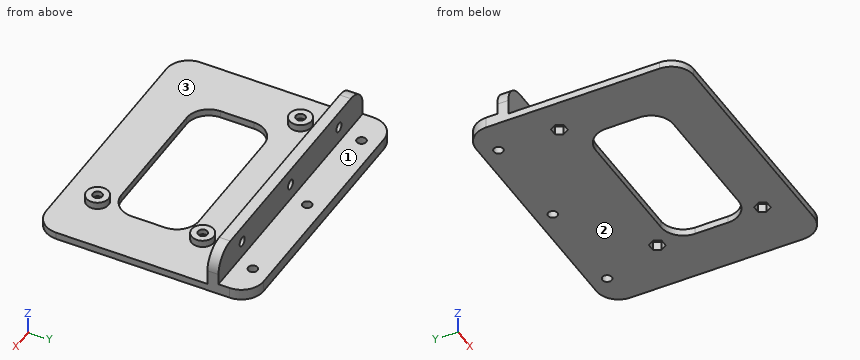
```python
from build123d import *

# Parameters (mm, degrees)
F0_W     = 121.6
F0_H     = 78.3
F0_R     = 2.125
F1_DEPTH = 3.2
F2_R     = 5
F2_R_2   = 2.125
F3_DEPTH = 3.2
F5_DEPTH = 4
F6_W     = 121.6
F6_H     = 20
F6_R     = 2.125
F7_DEPTH = 5
F8_W     = 121.6
F8_H     = 15
F8_R     = 2.125
F9_DEPTH = 5
F10_R    = 10


with BuildPart() as f1:
    # F0 (on Top) → F1 (new body)
    with BuildSketch(Plane.XY):
        Rectangle(F0_W, F0_H)
        with Locations((35.5, -24.05)):
            Circle(F0_R, mode=Mode.SUBTRACT)
        with BuildLine():
            ThreePointArc((37.5, -7.5), (34.571068, -14.571068), (27.5, -17.5))
            Line((27.5, -17.5), (-27.5, -17.5))
            ThreePointArc((-27.5, -17.5), (-34.571068, -14.571068), (-37.5, -7.5))
            Line((-37.5, -7.5), (-37.5, 7.5))
            ThreePointArc((-37.5, 7.5), (-34.571068, 14.571068), (-27.5, 17.5))
            Line((-27.5, 17.5), (27.5, 17.5))
            ThreePointArc((27.5, 17.5), (34.571068, 14.571068), (37.5, 7.5))
            Line((37.5, 7.5), (37.5, -7.5))
        make_face(mode=Mode.SUBTRACT)
        with Locations((-45.72, 24.15)):
            Circle(F0_R, mode=Mode.SUBTRACT)
        with Locations((36.8, 24.15)):
            Circle(F0_R, mode=Mode.SUBTRACT)
    extrude(amount=F1_DEPTH)

    # F2 (on face) → F3 (join)
    with BuildSketch(Plane.XY.offset(3.2)):
        with Locations((-45.72, 24.15)):
            Circle(F2_R)
        with Locations((-45.72, 24.15)):
            Circle(F2_R_2, mode=Mode.SUBTRACT)
        with Locations((36.8, 24.15)):
            Circle(F2_R)
        with Locations((36.8, 24.15)):
            Circle(F2_R_2, mode=Mode.SUBTRACT)
        with Locations((35.5, -24.05)):
            Circle(F2_R)
        with Locations((35.5, -24.05)):
            Circle(F2_R_2, mode=Mode.SUBTRACT)
    extrude(amount=F3_DEPTH)

    # F4 (on face) → F5 (cut)
    with BuildSketch(Plane(origin=(0, 0, 0), x_dir=(1, 0, 0), z_dir=(0, 0, -1))):
        Polygon((-44.03125, -21.225), (-47.40875, -21.225), (-49.097499, -24.15), (-47.40875, -27.075), (-44.03125, -27.075), (-42.342501, -24.15), align=None)
        Polygon((38.48875, -21.225), (35.11125, -21.225), (33.422501, -24.15), (35.11125, -27.075), (38.48875, -27.075), (40.177499, -24.15), align=None)
        Polygon((33.81125, 21.125), (37.18875, 21.125), (38.877499, 24.05), (37.18875, 26.975), (33.81125, 26.975), (32.122501, 24.05), align=None)
    extrude(amount=-F5_DEPTH, mode=Mode.SUBTRACT)

    # F6 (on Top) → F7 (join)
    with BuildSketch(Plane.XY):
        with Locations((0, 49.15)):
            Rectangle(F6_W, F6_H)
        with Locations((-45.8, 51.65)):
            Circle(F6_R, mode=Mode.SUBTRACT)
        with Locations((0, 51.65)):
            Circle(F6_R, mode=Mode.SUBTRACT)
        with Locations((45.8, 51.65)):
            Circle(F6_R, mode=Mode.SUBTRACT)
    extrude(amount=F7_DEPTH)

    # F8 (on face) → F9 (join)
    with BuildSketch(Plane.XZ.offset(-39.15)):
        with Locations((0, 12.5)):
            Rectangle(F8_W, F8_H)
        with Locations((-40.8, 12.5)):
            Circle(F8_R, mode=Mode.SUBTRACT)
        with Locations((0, 12.5)):
            Circle(F8_R, mode=Mode.SUBTRACT)
        with Locations((40.8, 12.5)):
            Circle(F8_R, mode=Mode.SUBTRACT)
    extrude(amount=-F9_DEPTH)

    # F10
    f10_edges = [f1.edges().sort_by_distance(p)[0] for p in [
        (60.8, -39.15, 1.6),
        (-60.8, -39.15, 1.6),
        (-60.8, 59.15, 2.5),
        (-60.8, 41.65, 20),
        (60.8, 41.65, 20),
        (60.8, 59.15, 2.5),
    ]]
    fillet(f10_edges, radius=F10_R)


solid = f1.part
```
Input: part model. Units: mm. Frame: model coordinates. Face numbers are marked on the shaded views. A direction names the side the tool comes from. Coordinates: 2 decimals unless noted, no trailing zeros. Order: outer loops, then holes, each group sorted by start corner. A loop starts at its lowest first (then second) coordinate and runs counter-clockwise, first axis right, second up. Notation, with made-up numbers: (24.5, 75) - (70.5, 75) arc R20 cw to (70.5, 105) - close; hole circle Ø10 at (44, 7.25). An arc over 180 degrees is marked (long way). Put each result on its own line as item: value.
1. Cut plane C-C on z = 12.5. Return the cut outline in (x, y) (3 decimals).
Report:
outline: (-60.482, 39.15) - (-42.925, 39.15) - (-42.925, 44.15) - (-60.482, 44.15) - close; (-38.675, 39.15) - (-2.125, 39.15) - (-2.125, 44.15) - (-38.675, 44.15) - close; (2.125, 39.15) - (38.675, 39.15) - (38.675, 44.15) - (2.125, 44.15) - close; (42.925, 39.15) - (60.482, 39.15) - (60.482, 44.15) - (42.925, 44.15) - close
2. Cut plane A-A on x = 19.5. Return the cut outline in (y, z).
Report:
outline: (-39.15, 0) - (-17.5, 0) - (-17.5, 3.2) - (-39.15, 3.2) - close; (17.5, 0) - (59.15, 0) - (59.15, 5) - (44.15, 5) - (44.15, 20) - (39.15, 20) - (39.15, 3.2) - (17.5, 3.2) - close
3. Cut plane D-D on y = 51.65. Return the cut outline in (x, z) (3 decimals), then the cut area to 3 significant figures.
Report:
outline: (-60.482, 0) - (-47.925, 0) - (-47.925, 5) - (-60.482, 5) - close; (-43.675, 0) - (-2.125, 0) - (-2.125, 5) - (-43.675, 5) - close; (2.125, 0) - (43.675, 0) - (43.675, 5) - (2.125, 5) - close; (47.925, 0) - (60.482, 0) - (60.482, 5) - (47.925, 5) - close
area: 541 mm2
4. Reachability of the marked faces 1, 2 and 3 from +Z, -Z, +X, -X, +Y, -Y: full face, straight path, thin tool, end or side. Return the list, or none.
Report:
face 1: +Z, +X, -X, +Y
face 2: -Z, +X, -X, +Y, -Y
face 3: +Z
5. Line query: line 1 along Y through (x, z) = (36, 4.5); line 2 along Z through (x, y) = (40.8, 40.7) (3 decimals); line 3 along Y through (x, z) = (-2.5, 1.25). Output: solid intervals per line, ascending.
Report:
line 1: y = -29.02 to -26.12, -21.98 to -19.08, 19.21 to 22.18, 26.12 to 29.09, 39.15 to 59.15
line 2: z = 0 to 10.375, 14.625 to 20
line 3: y = -39.15 to -17.5, 17.5 to 59.15
6. Contact query for flat-ended pins moving along their axis: pin 1 Ø4 at (x, y) = (-45.72, 24.15) entering from +Z; pin 2 Ø10 at (x, y) = (-45.5, -9.5) entering from +Z; pin 3 Ø1 at (x, y) = (9.5, 33.5) entering from -Z; pin 4 Ø3 at (x, y) = (36.5, -23) entering from +Z. Output: stop coordinate, or through.
Report:
pin 1: passes through
pin 2: stops at z = 3.2
pin 3: stops at z = 0
pin 4: stops at z = 6.4
7. Cut plane B-B on y = -0.5. Return the cut outline in (x, z), then the cut area to 3 significant figures.
Report:
outline: (-60.8, 0) - (-37.5, 0) - (-37.5, 3.2) - (-60.8, 3.2) - close; (37.5, 0) - (60.8, 0) - (60.8, 3.2) - (37.5, 3.2) - close
area: 149 mm2
